```python
from build123d import *

# Parameters (mm, degrees)
CROQUIS1_W              = 30
CROQUIS1_H              = 10
CROQUIS1_R              = 1.55
SALIENTE_EXTRUIR1_DEPTH = 4
CROQUIS2_R              = 2.8
CORTAR_EXTRUIR1_DEPTH   = 3
CROQUIS3_W              = 10
CROQUIS3_H              = 10
SALIENTE_EXTRUIR2_DEPTH = 10
CROQUIS4_R              = 2.6
CORTAR_EXTRUIR2_DEPTH   = 10
REDONDEO3_R             = 5


with BuildPart() as part:
    # Croquis1 → Saliente-Extruir1 (new body)
    with BuildSketch(Plane(origin=(0, 0, 0), x_dir=(1, 0, 0), z_dir=(0, 1, 0))):
        with Locations((15, 5)):
            Rectangle(CROQUIS1_W, CROQUIS1_H)
        with Locations(Location((5, 5, 0), (0, 0, 270))):
            Circle(CROQUIS1_R, mode=Mode.SUBTRACT)
        with Locations(Location((25, 5, 0), (0, 0, 270))):
            Circle(CROQUIS1_R, mode=Mode.SUBTRACT)
    extrude(amount=SALIENTE_EXTRUIR1_DEPTH)

    # Croquis2 → Cortar-Extruir1 (cut)
    with BuildSketch(Plane(origin=(0, 4, 0), x_dir=(1, 0, 0), z_dir=(0, 1, 0))):
        with Locations(Location((5, 5, 0), (0, 0, 270))):
            Circle(CROQUIS2_R)
        with Locations(Location((25, 5, 0), (0, 0, 270))):
            Circle(CROQUIS2_R)
    extrude(amount=-CORTAR_EXTRUIR1_DEPTH, mode=Mode.SUBTRACT)

    # Croquis3 → Saliente-Extruir2 (add)
    with BuildSketch(Plane(origin=(0, 4, 0), x_dir=(1, 0, 0), z_dir=(0, 1, 0))):
        with Locations((15, 5)):
            Rectangle(CROQUIS3_W, CROQUIS3_H)
    extrude(amount=SALIENTE_EXTRUIR2_DEPTH)

    # Croquis4 → Cortar-Extruir2 (cut)
    with BuildSketch(Plane.ZY.offset(-10)):
        with Locations((-5, 9)):
            Circle(CROQUIS4_R)
    extrude(amount=-CORTAR_EXTRUIR2_DEPTH, mode=Mode.SUBTRACT)

    # Redondeo3
    redondeo3_edges = [part.edges().sort_by_distance(p)[0] for p in [
        (15, 14, 0),
        (15, 14, -10),
    ]]
    fillet(redondeo3_edges, radius=REDONDEO3_R - 0.0001)  # a hair under: the kernel refuses the full size


solid = part.part
```
Geometry: final body of the model. Coordinates: model frame, mm. A direction names the side the tool comes from. Round coordinates to 2 decimals unless told otherwise and drop trailing zeros. Write each loop counter-clockwise with the first axis right and the second up, starting at its lowest first coordinate (ties: lowest second). Pieces come first, ordered by that corner, then holes. Notation, with made-up numbers: M 72,10 L 82,10 A18 ccw 82,29 Z; hole C 13,36.5 d3. An arc over 180 degrees is marked long. Answer in a Markdown table with one row per item. Add a question column.
(1) Ray query, L1, parallel to X at y = 0.75, z = -5; L2, parallel to X at y = 2.35, z = -5; L3, parallel to Z at x = 5, y = 0.35. Return the intervals inside material, ascending.
(2) Cut plane C-C, the plane z = -5.75. Return the cut outline in (x, y).
(3) Reachability of faces 1 (the face through (14.93, 6.46, -5.56)), 2 (the face through (27.36, 2.52, -3.49)), 3 (the face through (22.7, 4, -7.3)), 4 (the face through (30, 2, -5)), 5 (the face through (2.7, 4, -7.3)) from +Z, -Z, +X, -X, +Y, -Y: full face, straight path, thin tool, end or side. Return the list, or none.
(4) Contact query for flat-ended pins moving along their axis: pin 1 (2.5 mm diameter, centred on x = 25, z = -5, fed in from +Y); pin 2 (3 mm diameter, centred on x = 5, z = -4, fed in from +Y); pin 3 (3 mm diameter, centred on y = 11, z = -2.5, fed in from -X); pin 4 (1.5 mm diameter, centred on x = 19, z = -6, fed in from +Y). Output: stop coordinate, or through.
(5) Cut plane B-B, the plane y = 10.75. Return the cut outline in (x, z), then the cut area to 3 significant figures.
(6) Cut plane D-D, the plane y = 2.25. Return the cut outline in (x, z).
(7) Draft query along X for faces 6 (the face through (20, 7, -7)), 7 (the face through (15, 3, 0)), 8 (the face through (3.79, 1, -3.79)), 9 (the face through (0, 2, -5)). Return one class per face: pulls with the +X half, pulls with the -X half, needs draft (parallel to the pull), parting line crosses it, or undercut.
Established:
| question | item | result |
|---|---|---|
| 1 | L1 | 0 to 3.45, 6.55 to 23.45, 26.55 to 30 |
| 1 | L2 | 0 to 2.2, 7.8 to 22.2, 27.8 to 30 |
| 1 | L3 | -10 to -6.55, -3.45 to 0 |
| 2 | outline | M 0,0 L 3.64,0 L 3.64,1 L 2.3,1 L 2.3,4 L 0,4 Z; M 6.36,0 L 23.64,0 L 23.64,1 L 22.3,1 L 22.3,4 L 20,4 L 20,6.51 L 10,6.51 L 10,4 L 7.7,4 L 7.7,1 L 6.36,1 Z; M 10,11.49 L 20,11.49 L 20,13.94 L 10,13.94 Z; M 26.36,0 L 30,0 L 30,4 L 27.7,4 L 27.7,1 L 26.36,1 Z |
| 3 | face 1 | +X, -X |
| 3 | face 2 | +Y |
| 3 | face 3 | +Z, -Z, +X, +Y |
| 3 | face 4 | +Z, -Z, +X, +Y, -Y |
| 3 | face 5 | +Z, -Z, -X, +Y |
| 4 | pin 1 | through |
| 4 | pin 2 | y = 1 |
| 4 | pin 3 | x = 10 |
| 4 | pin 4 | y = 13.99 |
| 5 | outline | M 10,-9.68 L 20,-9.68 L 20,-6.92 L 10,-6.92 Z; M 10,-3.08 L 20,-3.08 L 20,-0.32 L 10,-0.32 Z |
| 5 | area | 55.2 mm² |
| 6 | outline | M 0,-10 L 30,-10 L 30,0 L 0,0 Z; hole C 5,-5 d5.6; hole C 25,-5 d5.6 |
| 7 | face 6 | pulls with the +X half |
| 7 | face 7 | needs draft |
| 7 | face 8 | undercut |
| 7 | face 9 | pulls with the -X half |
